from build123d import *

# Parameters (mm, degrees)
F0_R     = 15
F0_R_2   = 12.5
F0_R_3   = 10
F0_R_4   = 7
F1_DEPTH = 2
F2_DEPTH = 9
F3_R     = 15
F3_R_2   = 12.5
F3_R_3   = 10
F4_DEPTH = 2


# Not quite as in the source:
# - a fillet or chamfer that OpenCascade refuses, or shapes differently, is made with other operations: its cross-section is extruded or revolved along the edge and cut away or added


with BuildPart() as f1:
    # F0 (on Top) → F1 (new body)
    with BuildSketch(Plane.XY):
        Circle(F0_R)
        Circle(F0_R_2, mode=Mode.SUBTRACT)
        Circle(F0_R_2)
        Circle(F0_R_3, mode=Mode.SUBTRACT)
        Circle(F0_R_3)
        Circle(F0_R_4, mode=Mode.SUBTRACT)
    extrude(amount=F1_DEPTH)

    # F0 (on Top) → F2 (join)
    with BuildSketch(Plane.XY):
        Circle(F0_R_2)
        Circle(F0_R_3, mode=Mode.SUBTRACT)
    extrude(amount=F2_DEPTH)

    # F3 (on face) → F4 (join)
    with BuildSketch(Plane.XY.offset(9)):
        Circle(F3_R)
        Circle(F3_R_2, mode=Mode.SUBTRACT)
        Circle(F3_R_2)
        Circle(F3_R_3, mode=Mode.SUBTRACT)
    extrude(amount=F4_DEPTH)

    # F5: fillet of radius 3 on 2 edges, made by hand

    # F5_s1 → F5_t2 (revolve)
    with BuildSketch(Plane.XZ):
        with BuildLine():
            ThreePointArc((12.5, 4.9580398916), (13.2087121525, 3.0215482184), (15, 2))
            Line((15, 2), (12.5, 2))
            Line((12.5, 2), (12.5, 4.9580398916))
        make_face()
    revolve(axis=Axis((0, 0, 2), (0, 0, -1)))

    # F5_s3 → F5_t4 (revolve)
    with BuildSketch(Plane.XZ):
        with BuildLine():
            ThreePointArc((15, 9), (13.2087121525, 7.9784517816), (12.5, 6.0419601084))
            Line((12.5, 6.0419601084), (12.5, 9))
            Line((12.5, 9), (15, 9))
        make_face()
    revolve(axis=Axis((0, 0, 9), (0, 0, 1)))


solid = f1.part
Geometry: final body of the model. Coordinates: model frame, mm. A direction names the side the tool comes from. Round coordinates to 2 decimals unless told otherwise and drop trailing zeros. Order: outer loops, then holes, each group sorted by start corner. A loop starts at its lowest first (then second) coordinate and runs counter-clockwise, first axis right, second up. Notation, with made-up numbers: (39, 54) - (76, 54) arc R13 ccw to (76, 66) - close; hole circle Ø9 at (-10.5, 81). An arc over 180 degrees is marked (long way). Write each question's results on one line, items separated by ' | '.
Item 1: First-contact query: pin 1 Ø1 at (x, z) = (5.5, 9.5) entering from +Y; pin 2 Ø1 at (x, z) = (3, 2) entering from +Y; pin 3 Ø3 at (y, z) = (-5.5, 6) entering from -X. Flat tips, straight axial feed; report the tip coordinate or a pass-through.
Completed:
pin 1: y = 14.14 | pin 2: y = 14.79 | pin 3: x = -11.88
Item 2: Reachability of faces 1 (the flat face through (-7, -2, 2)), 2 (the cylindrical face through (-14.985, 0.66, 0.986)), 3 (the cylindrical face through (11.923, 3.755, 5.492)) from +Z, -Z, +X, -X, +Y, -Y: full face, straight path, thin tool, end or side. Return the list, or none.
Completed:
face 1: +Z | face 2: +Z, -Z | face 3: none
Item 3: Material intervals for line 1 along Y through (x, z) = (0, 0.95); line 2 along X through (y, z) = (-3.5, 4); line 3 along X through (y, z) = (-7.5, 3.5), sorted ascending. Write a range as [from, to].
Completed:
line 1: [-15, -7], [7, 15] | line 2: [-12.16, -9.37], [9.37, 12.16] | line 3: [-10.47, -6.61], [6.61, 10.47]
Item 4: Section C-C, the plane z = 4.25. Return the cut outline in (x, y).
Completed:
outline: circle Ø25.17 at (0, 0); hole circle Ø20 at (0, 0)
Item 5: Mould query, pull axis X, two halves, no side actions, for faces 4 (the cylindrical face through (-14.985, 0.66, 9.986)), 5 (the cylindrical face through (-2.17, -9.76, 6.44)), 6 (the flat face through (3.1, -6.5, 0)). Classes: pulls with the +X half, pulls with the -X half, needs draft (parallel to the pull), parting line crosses it, or undercut.
Completed:
face 4: parting line crosses it | face 5: undercut | face 6: needs draft
Item 6: Section A-A, the plane x = 0. Return the cut outline in (y, z), and give its area (3 significant figures).
Completed:
outline: (-15, 0) - (-7, 0) - (-7, 2) - (-10, 2) - (-10, 11) - (-15, 11) - (-15, 9) arc R3 cw to (-12.5, 6.04) - (-12.5, 4.96) arc R3 cw to (-15, 2) - close; (7, 0) - (15, 0) - (15, 2) arc R3 cw to (12.5, 4.96) - (12.5, 6.04) arc R3 cw to (15, 9) - (15, 11) - (10, 11) - (10, 2) - (7, 2) - close | area: 94.3 mm^2
